Model file for the job. Use its own axes, mm. Face numbers are marked on the shaded views. Round coordinates to 2 decimals unless told otherwise and drop trailing zeros. Loops run counter-clockwise (first coordinate to the right, second up) from the corner with the lowest first, then second, coordinate; pieces in that order, holes last. Notation, with made-up numbers: (-1, 15.25) - (40, 15.25) arc R21 ccw to (40, 53.25) - close; hole circle Ø7 at (-7.75, -15.75). An arc over 180 degrees is marked (long way). Use one line per item in the form item = value.
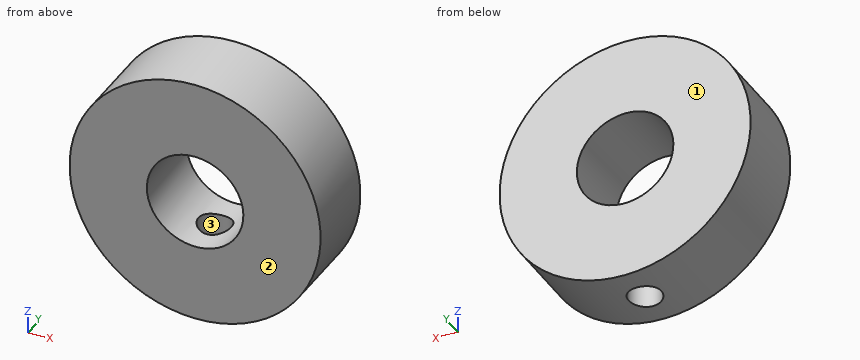
from build123d import *

# Parameters (mm, degrees)
SKETCH1_R           = 6.5
BOSS_EXTRUDE1_DEPTH = 4
SKETCH2_R           = 2.5
CUT_EXTRUDE1_DEPTH  = 11.024968828
SKETCH3_R           = 0.85
CUT_EXTRUDE2_DEPTH  = 11.024968828


with BuildPart() as part:
    # Sketch1 → Boss-Extrude1 (new body)
    with BuildSketch(Plane(origin=(0, 0, 0), x_dir=(1, 0, 0), z_dir=(0, 1, 0))):
        with Locations(Location((0, 0, 0), (0, 0, 270))):
            Circle(SKETCH1_R)
    extrude(amount=BOSS_EXTRUDE1_DEPTH)

    # Sketch2 → Cut-Extrude1 (cut, through all)
    with BuildSketch(Plane(origin=(0, 4, 0), x_dir=(1, 0, 0), z_dir=(0, 1, 0))):
        with Locations(Location((0, 0, 0), (0, 0, 270))):
            Circle(SKETCH2_R)
    extrude(amount=-CUT_EXTRUDE1_DEPTH, mode=Mode.SUBTRACT)

    # Sketch3 → Cut-Extrude2 (cut, through all)
    with BuildSketch(Plane.XY):
        with Locations((0, 2)):
            Circle(SKETCH3_R)
    extrude(amount=-CUT_EXTRUDE2_DEPTH, mode=Mode.SUBTRACT)


solid = part.part
1. Cut at A-A, the plane z = 0. Give the cut face in (x, y), plus the area to 3 significant figures.
Geometry check:
outline = (-6.5, 0) - (-2.5, 0) - (-2.5, 4) - (-6.5, 4) - close; (2.5, 0) - (6.5, 0) - (6.5, 4) - (2.5, 4) - close
area = 32.0 mm^2
2. Cut at B-B, the plane x = 0. Give the cut face in (y, z), plus the area to 3 significant figures.
Geometry check:
outline = (0, -6.5) - (1.15, -6.5) - (1.15, -2.5) - (0, -2.5) - close; (0, 2.5) - (4, 2.5) - (4, 6.5) - (0, 6.5) - close; (2.85, -6.5) - (4, -6.5) - (4, -2.5) - (2.85, -2.5) - close
area = 25.2 mm^2
3. Flat gauge pins, fed straight in: pin 1 (2 mm diameter, centred on y = 3, z = 1.5, fed in from -X); pin 2 (4.5 mm diameter, centred on x = 0, z = 0, fed in from +Y); pin 3 (5 mm diameter, centred on x = 1.5, z = 2, fed in from -Y); pin 4 (1.5 mm diameter, centred on x = 0, y = 2, fed in from -Z). Where does each tip first touch, or does it go through?
Geometry check:
pin_1 = -6.48
pin_2 = through
pin_3 = 0
pin_4 = 2.38
4. Cut at D-D, the plane z = -5.25. Give the cut face in (x, y).
Geometry check:
outline = (-3.83, 0) - (3.83, 0) - (3.83, 4) - (-3.83, 4) - close; hole circle Ø1.7 at (0, 2)
5. Pull direction Y, two halves, no side cores. Call the marked faces 1, 2 and 3: +Y half, -Y half, draft (parallel to the pull), parting line (faces both ways), or undercut.
Geometry check:
face_1 = +Y half
face_2 = -Y half
face_3 = undercut
6. Cut at C-C, the plane y = 3.35. Give the cut face in (x, z).
Geometry check:
outline = circle Ø13 at (0, 0); hole circle Ø5 at (0, 0)
7. Wall check: probe 1 along X at (y, z) = (1.4, 0); probe 2 along Z at (x, y) = (0, 1.55). Give the ranges that are in metal, low to high.
Geometry check:
probe_1 = -6.5 to -2.5, 2.5 to 6.5
probe_2 = 2.5 to 6.5
